```python
from build123d import *

# Parameters (mm, degrees)
SKETCH1_R           = 4.4
BOSS_EXTRUDE1_DEPTH = 4
BOSS_EXTRUDE2_DEPTH = 9
SKETCH3_R           = 2.3
CUT_EXTRUDE1_DEPTH  = 13


with BuildPart() as part:
    # Sketch1 → Boss-Extrude1 (new body)
    with BuildSketch(Plane(origin=(0, 0, 0), x_dir=(1, 0, 0), z_dir=(0, 1, 0))):
        with BuildLine():
            Line((-67, 35), (67, 35))
            ThreePointArc((67, 35), (72.656854249, 32.656854249), (75, 27))
            Line((75, 27), (75, -27))
            ThreePointArc((75, -27), (72.656854249, -32.656854249), (67, -35))
            Line((67, -35), (-67, -35))
            ThreePointArc((-67, -35), (-72.656854249, -32.656854249), (-75, -27))
            Line((-75, -27), (-75, 27))
            ThreePointArc((-75, 27), (-72.656854249, 32.656854249), (-67, 35))
        make_face()
        with Locations((-45, -17.5)):
            Circle(SKETCH1_R, mode=Mode.SUBTRACT)
        with Locations((45, -17.5)):
            Circle(SKETCH1_R, mode=Mode.SUBTRACT)
    extrude(amount=-BOSS_EXTRUDE1_DEPTH)

    # Sketch2 → Boss-Extrude2 (add)
    with BuildSketch(Plane(origin=(0, 0, 0), x_dir=(1, 0, 0), z_dir=(0, 1, 0))):
        with BuildLine():
            Line((-75, 5), (75, 5))
            Line((75, 5), (75, 27))
            ThreePointArc((75, 27), (72.656854249, 32.656854249), (67, 35))
            Line((67, 35), (-67, 35))
            ThreePointArc((-67, 35), (-72.656854249, 32.656854249), (-75, 27))
            Line((-75, 27), (-75, 5))
        make_face()
    extrude(amount=BOSS_EXTRUDE2_DEPTH)

    # Sketch3 → Cut-Extrude1 (cut)
    with BuildSketch(Plane(origin=(0, 9, 0), x_dir=(1, 0, 0), z_dir=(0, 1, 0))):
        with Locations((-54, 20)):
            Circle(SKETCH3_R)
        with Locations((-27, 20)):
            Circle(SKETCH3_R)
        with Locations((0, 20)):
            Circle(SKETCH3_R)
        with Locations((27, 20)):
            Circle(SKETCH3_R)
        with Locations((54, 20)):
            Circle(SKETCH3_R)
    extrude(amount=-CUT_EXTRUDE1_DEPTH, mode=Mode.SUBTRACT)


solid = part.part
```
Geometry check sheet. Reference: the model listing, model coordinates, mm. A direction names the side the tool comes from. Coordinates: 2 decimals unless noted, no trailing zeros. Loops run counter-clockwise (first coordinate to the right, second up) from the corner with the lowest first, then second, coordinate; pieces in that order, holes last.
Item 1: Sectioned sample at C-C, the plane y = 6. Record the boundary of the cut face in (x, z), then the cut area to 3 significant figures.
Item 2: Go/stop test with flat-tipped pins: pin 1 Ø10 at (x, z) = (45, 17.5) entering from -Y; pin 2 Ø1.5 at (x, y) = (-45.5, 3.5) entering from +Z; pin 3 Ø20 at (x, z) = (33, 19.5) entering from +Y; pin 4 Ø3.5 at (x, z) = (54, -20) entering from -Y. Record where each tip stops, or that it passes through.
Item 3: Sectioned sample at A-A, the plane x = 45. Record the boundary of the cut face in (y, z).
Item 4: Sectioned sample at B-B, the plane z = 17.5. Record the boundary of the cut face in (x, y).
Item 5: Release check for a two-part mould opening along Z. For faces 1 (the face through (26.501, 2.591, -17.755)), 2 (the face through (1, 2, -35)), 3 (the face through (1, -4, 0)) record: released by +Z, released by -Z, zero draft, split by the parting line, or undercut.
Item 6: Access from +Z, -Z, +X, -X, +Y, -Y to the whole of each face (thin tool, end or side, straight path). Record for faces 4 (the face through (47.365, -1.972, 13.79)), 5 (the face through (-1, 4, -5)).
Item 7: Sectioned sample at D-D, the plane x = -54. Record the boundary of the cut face in (y, z), then the cut area to 3 significant figures.
Item 8: Thickness scan on line 1 (X direction, y = 7.75, z = -20); line 2 (X direction, y = -2.65, z = 17.5); line 3 (Z direction, x = 27, y = 6.5). Record the ranges inside material, lowest first.
Check result:
1. outline: (-75, -27) arc R8 ccw to (-67, -35) - (67, -35) arc R8 ccw to (75, -27) - (75, -5) - (-75, -5) - close; hole circle Ø4.6 at (-54, -20); hole circle Ø4.6 at (-27, -20); hole circle Ø4.6 at (0, -20); hole circle Ø4.6 at (27, -20); hole circle Ø4.6 at (54, -20)
1. area: 4,390 mm2
2. pin 1: stops at y = -4
2. pin 2: stops at z = -5
2. pin 3: stops at y = 0
2. pin 4: passes through
3. outline: (-4, -35) - (9, -35) - (9, -5) - (0, -5) - (0, 13.1) - (-4, 13.1) - close; (-4, 21.9) - (0, 21.9) - (0, 35) - (-4, 35) - close
4. outline: (-75, -4) - (-49.4, -4) - (-49.4, 0) - (-75, 0) - close; (-40.6, -4) - (40.6, -4) - (40.6, 0) - (-40.6, 0) - close; (49.4, -4) - (75, -4) - (75, 0) - (49.4, 0) - close
5. face 1: undercut
5. face 2: released by -Z
5. face 3: zero draft
6. face 4: +Y, -Y
6. face 5: +Z, +X, -X, +Y
7. outline: (-4, -35) - (9, -35) - (9, -22.3) - (-4, -22.3) - close; (-4, -17.7) - (9, -17.7) - (9, -5) - (0, -5) - (0, 35) - (-4, 35) - close
7. area: 490 mm2
8. line 1: x = -75 to -56.3, -51.7 to -29.3, -24.7 to -2.3, 2.3 to 24.7, 29.3 to 51.7, 56.3 to 75
8. line 2: x = -75 to -49.4, -40.6 to 40.6, 49.4 to 75
8. line 3: z = -35 to -22.3, -17.7 to -5
